Read the model definition and answer for the solid it produces. Units are mm, in the model's axes. Face numbers are marked on the shaded views. Coordinates: 2 decimals unless noted, no trailing zeros. Write each loop counter-clockwise with the first axis right and the second up, starting at its lowest first coordinate (ties: lowest second). Pieces come first, ordered by that corner, then holes.
(1) Find the intervals of material crossed by probe 1 along Z at (x, y) = (3, -16); probe 2 along Y at (x, z) = (0.5, -5.5); probe 3 along Y at (x, z) = (-4, 2.5), in increasing order.
(2) Section B-B on y = 0 is taken. Write down the section's boundary in (x, z).
(3) The mould has two halves that part along X. Classify the marked faces 1, 2 and 3: +X half, -X half, draft (parallel to the pull), parting line (faces both ways), or undercut.
(4) Section C-C on z = 2 is taken. Write down the section's boundary in (x, y), then the cut area to 3 significant figures.
(5) Given pin 1 (3.5 mm diameter, centred on x = 1, y = 8, fed in from -Z); pin 2 (5.5 mm diameter, centred on y = -15.875, z = 3.937, fed in from -X); pin 3 (3 mm diameter, centred on x = 0, y = 8.74, fed in from -Z), each flat-ended and moving along its own axis, determine where each tip first touches the part or whether it passes through.
(6) Section A-A on x = 0 is taken. State how many separate pieces and enclosed holes the cut face has, then the cut area to 3 significant figures.
from build123d import *

# Parameters (mm, degrees)
SKETCH1_W                                          = 31.75
SKETCH1_H                                          = 32.1564
BOSS_EXTRUDE1_DEPTH                                = 9.525
SKETCH2_W                                          = 8.763
SKETCH2_H                                          = 32.1564
CUT_EXTRUDE1_DEPTH                                 = 27.563955842
CUT_EXTRUDE2_DEPTH                                 = 27.563955842
SKETCH4_W                                          = 8.763
SKETCH4_H                                          = 32.16
CUT_EXTRUDE3_DEPTH                                 = 27.563955842
SKETCH5_W                                          = 9.525
SKETCH5_H                                          = 4.7625
SKETCH6_W                                          = 1.3208
SKETCH6_H                                          = 6.1087
CBORE_FOR_M3_5_HEX_HEAD_MACHINE_SCREW1_D           = 3.9116
CBORE_FOR_M3_5_HEX_HEAD_MACHINE_SCREW1_DEPTH       = 14.224
CBORE_FOR_M3_5_HEX_HEAD_MACHINE_SCREW1_CBORE_D     = 7.1374
CBORE_FOR_M3_5_HEX_HEAD_MACHINE_SCREW1_CBORE_DEPTH = 3.9116
M4_CLEARANCE_HOLE1_D                               = 4.572


with BuildPart() as part:
    # Sketch1 → Boss-Extrude1 (new body)
    with BuildSketch(Plane(origin=(4.7625, 0, 0), x_dir=(0, 0, -1), z_dir=(1, 0, 0))):
        with Locations((0, -2.9718)):
            Rectangle(SKETCH1_W, SKETCH1_H)
    extrude(amount=-BOSS_EXTRUDE1_DEPTH)

    # Sketch2 → Cut-Extrude1 (cut, through all)
    with BuildSketch(Plane.ZY.offset(4.7625)):
        with Locations((-11.4935, -2.9718)):
            Rectangle(SKETCH2_W, SKETCH2_H)
    extrude(amount=-CUT_EXTRUDE1_DEPTH, mode=Mode.SUBTRACT)

    # Sketch3 → Cut-Extrude2 (cut, through all)
    with BuildSketch(Plane.ZY.offset(4.7625)):
        with BuildLine():
            Line((1.0033, 13.1064), (-1.0033, 13.1064))
            Line((-1.0033, 13.1064), (-1.0033, 4.655619761))
            ThreePointArc((-1.0033, 4.655619761), (0, 4.7625), (1.0033, 4.655619761))
            Line((1.0033, 4.655619761), (1.0033, 13.1064))
        make_face()
    extrude(amount=-CUT_EXTRUDE2_DEPTH, mode=Mode.SUBTRACT)

    # Sketch4 → Cut-Extrude3 (cut, through all)
    with BuildSketch(Plane.ZY.offset(4.7625)):
        with Locations((11.4935, -2.9736)):
            Rectangle(SKETCH4_W, SKETCH4_H)
    extrude(amount=-CUT_EXTRUDE3_DEPTH, mode=Mode.SUBTRACT)

    # Sketch5 → Cut-Revolve1 (revolve, cut)
    with BuildSketch(Plane.XY):
        with Locations((0, 2.38125)):
            Rectangle(SKETCH5_W, SKETCH5_H)
    revolve(axis=Axis((-4.7625, 0, 0), (1, 0, 0)), mode=Mode.SUBTRACT)

    # Sketch6 → Hole1 (revolve, cut)
    with BuildSketch(Plane(origin=(0, 8.7376, 1.0033), x_dir=(0, 1, 0), z_dir=(1, 0, 0))):
        with Locations((0.6604, 3.05435)):
            Rectangle(SKETCH6_W, SKETCH6_H)
    revolve(axis=Axis((0, 8.7376, 111.0033), (0, 0, -1)), mode=Mode.SUBTRACT)

    # CBORE for M3.5 Hex Head Machine Screw1
    with Locations(Plane(origin=(0, 0, -7.112), x_dir=(-1, 0, 0), z_dir=(0, 0, -1))):
        with Locations((0, 8.7376)):
            CounterBoreHole(CBORE_FOR_M3_5_HEX_HEAD_MACHINE_SCREW1_D / 2, CBORE_FOR_M3_5_HEX_HEAD_MACHINE_SCREW1_CBORE_D / 2, CBORE_FOR_M3_5_HEX_HEAD_MACHINE_SCREW1_CBORE_DEPTH, depth=CBORE_FOR_M3_5_HEX_HEAD_MACHINE_SCREW1_DEPTH)

    # M4 Clearance Hole1 (through all)
    with Locations(Plane(origin=(4.7625, -17.4625, 0), x_dir=(0, 1, 0), z_dir=(1, 0, 0))):
        with Locations((1.5875, -3.937), (1.5875, 3.937)):
            Hole(M4_CLEARANCE_HOLE1_D / 2)


solid = part.part
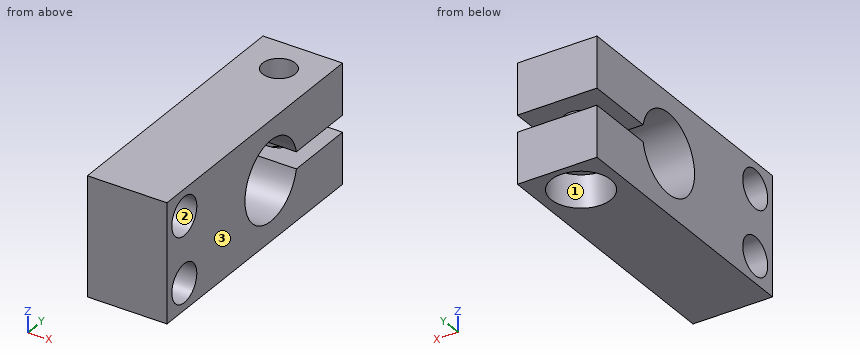
Response:
1. probe 1: z = -7.11 to -6.22, -1.65 to 1.65, 6.22 to 7.11
1. probe 2: y = -19.05 to -17.54, -14.21 to 5.2, 12.27 to 13.11
1. probe 3: y = -19.05 to -17.65, -14.1 to -4.05, 4.05 to 13.11
2. outline: (-4.76, -7.11) - (4.76, -7.11) - (4.76, -4.76) - (-4.76, -4.76) - close; (-4.76, 4.76) - (4.76, 4.76) - (4.76, 7.11) - (-4.76, 7.11) - close
3. face 1: undercut
3. face 2: draft
3. face 3: +X half
4. outline: (-4.76, -19.05) - (4.76, -19.05) - (4.76, -17.09) - (-4.76, -17.09) - close; (-4.76, -14.66) - (4.76, -14.66) - (4.76, -4.32) - (-4.76, -4.32) - close; (-4.76, 4.32) - (4.76, 4.32) - (4.76, 13.11) - (-4.76, 13.11) - close; hole circle Ø3.91 at (0, 8.74)
4. area: 189 mm2
5. pin 1: stops at z = -3.2
5. pin 2: stops at x = -4.76
5. pin 3: passes through
6. separate pieces: 3
6. enclosed holes: 2
6. area: 276 mm2
